Verification items for the finished model (mm, model axes). Round coordinates to 2 decimals unless told otherwise and drop trailing zeros. Order: outer loops, then holes, each group sorted by start corner. A loop starts at its lowest first (then second) coordinate and runs counter-clockwise, first axis right, second up. Notation, with made-up numbers: (27.25, 60) -> (67.25, 60) arc R13 cw to (67.25, 64) -> close; hole circle Ø1 at (4, -6.5). An arc over 180 degrees is marked (long way). Answer in a Markdown table with one row per item. Add a question column.
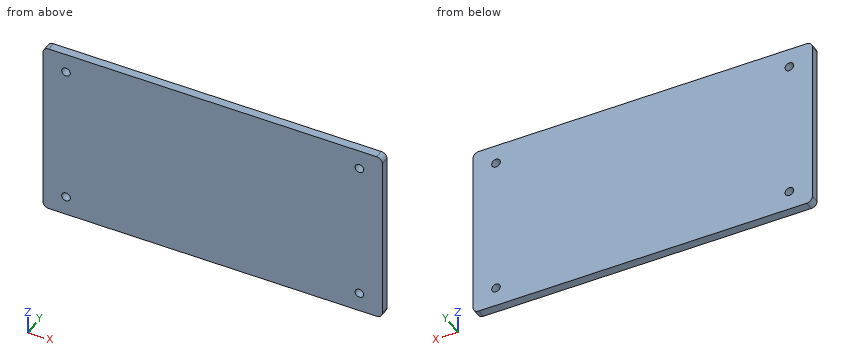
Autodesk Inventor part; units mm, degrees
ref_plane "YZ Plane" through (0, 0, 0) normal (1, 0, 0) x (0, 1, 0)
ref_plane "XZ Plane" through (0, 0, 0) normal (0, 1, 0) x (-1, 0, 0)
ref_plane "XY Plane" through (0, 0, 0) normal (0, 0, 1) x (1, 0, 0)
sketch "Sketch1" plane through (0, 0, 0) normal (0, 1, 0) x (-1, 0, 0)
  line L0 (0, 0) -> (150, 0)
  line L1 (150, 0) -> (150, -140)
  line L2 (150, -140) -> (0, -140)
  line L3 (0, -140) -> (0, 0)
  line L4 (150, -70) -> (0, -70) construction
  line L5 (24, -45.75) -> (126, -45.75) construction
  line L6 (126, -45.75) -> (126, -94.25) construction
  line L7 (126, -94.25) -> (24, -94.25) construction
  line L8 (24, -94.25) -> (24, -45.75) construction
  line L9 (24, -45.75) -> (126, -94.25) construction
  line L10 (126, -45.75) -> (24, -94.25) construction
  circle A0 centre (126, -45.75) radius 1.5
  circle A1 centre (126, -94.25) radius 1.5
  circle A2 centre (24, -94.25) radius 1.5
  circle A3 centre (24, -45.75) radius 1.5
  point P0 (75, -70)
  dimension "d0" = 150
  dimension "d1" = 140
  dimension "d2" = 102
  dimension "d3" = 48.5
  dimension "d4" = 3
  dimension "d5" = 3
  dimension "d6" = 3
  dimension "d7" = 3
extrude "Extrusion1" add sketch "Sketch1" along normal blind 3
sketch "Sketch2" plane through (0, 3, 0) normal (0, 1, 0) x (1, 0, 0)
  line L0 (-150, 140) -> (-150, 0)
  line L1 (-150, 50) -> (-147, 50)
  line L2 (-147, 50) -> (-147, 90)
  line L3 (-147, 90) -> (-150, 90)
  line L4 (-150, 90) -> (-150, 50)
  line L5 (-147, 70) -> (-150, 70) construction
  line L6 (0, 0) -> (0, 140)
  line L7 (0, 70) -> (-150, 70) construction
  line L8 (-150, 0) -> (0, 0)
  line L9 (-75, 0) -> (-75, 98) construction
  line L10 (-95, 0) -> (-55, 0)
  line L11 (-55, 0) -> (-55, 3)
  line L12 (-55, 3) -> (-95, 3)
  line L13 (-95, 3) -> (-95, 0)
  line L14 (-75, 3) -> (-75, 0) construction
  line L15 (0, 50) -> (-3, 50)
  line L16 (-3, 50) -> (-3, 90)
  line L17 (-3, 90) -> (0, 90)
  line L18 (0, 90) -> (0, 50)
  line L19 (-3, 70) -> (0, 70) construction
  line L20 (-95, 140) -> (-55, 140)
  line L21 (-55, 140) -> (-55, 137)
  line L22 (-55, 137) -> (-95, 137)
  line L23 (-95, 137) -> (-95, 140)
  line L24 (-75, 137) -> (-75, 140) construction
  point P0 (0, 50)
  point P1 (0, 90)
  point P2 (-55, 0)
  dimension "d10" = 40
  dimension "d11" = 3
  dimension "d12" = 40
  dimension "d13" = 3
extrude "Extrusion2" cut sketch "Sketch2" against normal blind 5
sketch "Sketch3" plane through (0, 3, 0) normal (0, 1, 0) x (1, 0, 0)
  line L0 (-147, 50) -> (-147, 90)
  line L1 (-147, 70) -> (-3, 70) construction
  line L2 (-3, 50) -> (-3, 90)
  line L3 (-134, 39) -> (-16, 39)
  line L4 (-16, 39) -> (-16, 101)
  line L5 (-16, 101) -> (-134, 101)
  line L6 (-134, 101) -> (-134, 39)
  line L7 (-134, 39) -> (-16, 101) construction
  line L8 (-16, 39) -> (-134, 101) construction
  point P0 (0, 0)
  point P1 (-75, 70)
  dimension "d16" = 118
  dimension "d17" = 62
extrude "Extrusion3" cut sketch "Sketch3" against normal blind 10 keep common part
fillet "Fillet1" radius 2 4 edges at (-16, 1.5, -39) (-16, 1.5, -101) (-134, 1.5, -39) (-134, 1.5, -101)
properties part number "Spacer"
1) Cross-section at B-B, the plane z = -94.25. Record the boundary of the cut face in (x, y).
2) Thickness scan on L1, parallel to Z at x = -24, y = 2.4; L2, parallel to X at y = 1.85, z = -94.25; L3, parallel to X at y = 0.45, z = -95. Record the ranges inside material, lowest first. Write a range as [from, to].
3) Depth check by flat-ended pin: P1, Ø4, axis at x = -24, z = -45.75, coming from the -Y side. Enter the tip coordinate at first touch or a pass-through.
4) Cross-section at A-A, the plane x = -126. Record the boundary of the cut face in (y, z), and give its area (3 significant figures).
Results below:
| question | item | result |
|---|---|---|
| 1 | outline | (-134, 0) -> (-127.5, 0) -> (-127.5, 3) -> (-134, 3) -> close; (-124.5, 0) -> (-25.5, 0) -> (-25.5, 3) -> (-124.5, 3) -> close; (-22.5, 0) -> (-16, 0) -> (-16, 3) -> (-22.5, 3) -> close |
| 2 | L1 | [-101, -95.75], [-92.75, -47.25], [-44.25, -39] |
| 2 | L2 | [-134, -127.5], [-124.5, -25.5], [-22.5, -16] |
| 2 | L3 | [-134, -127.3], [-124.7, -25.3], [-22.7, -16] |
| 3 | P1 | y = 0 |
| 4 | outline | (0, -101) -> (3, -101) -> (3, -95.75) -> (0, -95.75) -> close; (0, -92.75) -> (3, -92.75) -> (3, -47.25) -> (0, -47.25) -> close; (0, -44.25) -> (3, -44.25) -> (3, -39) -> (0, -39) -> close |
| 4 | area | 168 mm² |
